Geometry: final body of the model. Coordinates: model frame, mm. A direction names the side the tool comes from. Give positions to 0.01 mm unless a question says otherwise; leave off trailing zeros. Write each loop counter-clockwise with the first axis right and the second up, starting at its lowest first coordinate (ties: lowest second). Pieces come first, ordered by that corner, then holes.
Q1. Section D-D (y = 1). Return the cut outline in (x, z), plus the area to 3 significant figures.
Q2. Line query: line 1 (Z direction, x = 175.5, y = -18.5); line 2 (X direction, y = -15, z = -9); line 3 (X direction, y = -11, z = -8). Output: solid intervals per line, ascending.
Q3. Section C-C (y = -16). Return the cut outline in (x, z).
Q4. Section A-A (x = 85). Return the cut outline in (y, z).
Q5. Pin query (flat end, axial travel): pin 1 Ø4 at (x, y) = (148.5, -0.5) entering from -Z; pin 2 Ø8 at (x, z) = (66.5, 9) entering from +Y; pin 3 Ø8.5 at (x, z) = (89.5, 5.5) entering from +Y. Return the tip coordinate at first contact, or that it passes through.
Q6. Mould query, pull axis Z, two halves, no side actions, for faces 5 (the flat face through (112, -10, -15)), 6 (the flat face through (0, -14, 0)), 7 (the flat face through (112, -12, -14)). Classes: +Z half, -Z half, draft (parallel to the pull), parting line (faces both ways), or undercut.
Q7. Reachability of faces 1 (the flat face through (0, 14, 0)), 2 (the flat face through (208, 9, 0)), 3 (the flat face through (0, 0, -14)), 4 (the cylindrical face through (114, 1, 3)) from +Z, -Z, +X, -X, +Y, -Y: full face, straight path, thin tool, end or side. Return the list, or none.
Q8. Section B-B (z = 0). Return the cut outline in (x, y).
from build123d import *

# Parameters (mm, degrees)
SKETCH_1_W         = 30
SKETCH_1_H         = 28
EXTRUDE_1_DEPTH    = 14
SKETCH_2_W         = 30
SKETCH_2_H         = 34
EXTRUDE_2_DEPTH    = 5.5
EXTRUDE_3_DEPTH    = 185
SKETCH_4_W         = 30
SKETCH_4_H         = 28
EXTRUDE_4_DEPTH    = 5.5
SKETCH_5_R         = 3
EXTRUDE_5_DEPTH    = 190.5
SKETCH1_R          = 1.5
CUT_EXTRUDE1_DEPTH = 10


with BuildPart() as part:
    # 草图1 → 凸台-拉伸1 (new body, symmetric)
    with BuildSketch(Plane.XY):
        Rectangle(SKETCH_1_W, SKETCH_1_H)
    extrude(amount=EXTRUDE_1_DEPTH, both=True)

    # 草图2 → 凸台-拉伸2 (add)
    with BuildSketch(Plane(origin=(15, 0, 0), x_dir=(0, 0, -1), z_dir=(1, 0, 0))):
        with Locations((0, -2)):
            Rectangle(SKETCH_2_W, SKETCH_2_H)
    extrude(amount=EXTRUDE_2_DEPTH)

    # 草图3 → 凸台-拉伸3 (add)
    with BuildSketch(Plane(origin=(20.5, 0, 0), x_dir=(0, 0, -1), z_dir=(1, 0, 0))):
        Polygon((-15, -19), (15, -19), (15, -6), (14, -6), (14, -18), (-14, -18), (-14, -6), (-15, -6), align=None)
    extrude(amount=EXTRUDE_3_DEPTH)

    # 草图4 → 凸台-拉伸4 (add)
    with BuildSketch(Plane(origin=(205.5, 0, 0), x_dir=(0, 0, -1), z_dir=(1, 0, 0))):
        with Locations((0, -5)):
            Rectangle(SKETCH_4_W, SKETCH_4_H)
    extrude(amount=EXTRUDE_4_DEPTH)

    # 草图5 → 凸台-拉伸5 (add)
    with BuildSketch(Plane(origin=(211, 0, 0), x_dir=(0, 0, -1), z_dir=(1, 0, 0))):
        with Locations((0, 1)):
            Circle(SKETCH_5_R)
    extrude(amount=-EXTRUDE_5_DEPTH)

    # Sketch1 → Cut-Extrude1 (cut)
    with BuildSketch(Plane.XZ.offset(19)):
        with Locations((50.5, 8.5)):
            Circle(SKETCH1_R)
        with Locations((175.5, 8.5)):
            Circle(SKETCH1_R)
        with Locations((175.5, -8.5)):
            Circle(SKETCH1_R)
        with Locations((50.5, -8.5)):
            Circle(SKETCH1_R)
    extrude(amount=-CUT_EXTRUDE1_DEPTH, mode=Mode.SUBTRACT)


solid = part.part
Computed:
1. outline: (-15, -14) - (15, -14) - (15, -15) - (20.5, -15) - (20.5, -3) - (205.5, -3) - (205.5, -15) - (211, -15) - (211, 15) - (205.5, 15) - (205.5, 3) - (20.5, 3) - (20.5, 15) - (15, 15) - (15, 14) - (-15, 14) - close
1. area: 2,280 mm2
2. line 1: z = -15 to -10, -7 to 7, 10 to 15
2. line 2: x = 15 to 20.5, 205.5 to 211
2. line 3: x = -15 to 20.5, 205.5 to 211
3. outline: (15, -15) - (211, -15) - (211, 15) - (15, 15) - close; hole (20.5, -14) - (205.5, -14) - (205.5, 14) - (20.5, 14) - close
4. outline: (-19, -15) - (-6, -15) - (-6, -14) - (-18, -14) - (-18, 14) - (-6, 14) - (-6, 15) - (-19, 15) - close; circle Ø6 at (1, 0)
5. pin 1: stops at z = -3
5. pin 2: stops at y = -18
5. pin 3: stops at y = 3.73
6. face 5: -Z half
6. face 6: draft
6. face 7: undercut
7. face 1: +Z, -Z, -X, +Y
7. face 2: +Z, -Z, +X, +Y
7. face 3: -Z, -X, +Y, -Y
7. face 4: none
8. outline: (-15, -14) - (15, -14) - (15, -19) - (211, -19) - (211, 9) - (205.5, 9) - (205.5, 4) - (20.5, 4) - (20.5, 15) - (15, 15) - (15, 14) - (-15, 14) - close; hole (20.5, -18) - (205.5, -18) - (205.5, -2) - (20.5, -2) - close
